```python
from build123d import *

# Parameters (mm, degrees)
FILLET1_R   = 0.2
HEX_2_DEPTH = 1.9


with BuildPart() as part:
    # BodySke → BaseBody (revolve)
    with BuildSketch(Plane.XY):
        Polygon((0, 0), (0, 4.715), (0.885, 4.715), (3.1, 2.5), (15.555, 2.5), (16, 2.055), (16, 0), align=None)
    revolve(axis=Axis((0, 0, 0), (1, 0, 0)))

    # Fillet1
    fillet1_edges = [part.edges().sort_by_distance(p)[0] for p in [
        (3.1, -2.5, 0),
    ]]
    fillet(fillet1_edges, radius=FILLET1_R)

    # Sketch2 → PreBroach (revolve, cut)
    with BuildSketch(Plane.XY):
        Polygon((0, 1.5), (1.9, 1.5), (2.766025404, 0), (0, 0), align=None)
    revolve(axis=Axis((0, 0, 0), (1, 0, 0)), mode=Mode.SUBTRACT)

    # Sketch3 → Hex 2 (cut)
    with BuildSketch(Plane.ZY):
        Polygon((-1.5, -0.866025404), (-1.5, 0.866025404), (0, 1.732050808), (1.5, 0.866025404), (1.5, -0.866025404), (0, -1.732050808), align=None)
    extrude(amount=-HEX_2_DEPTH, mode=Mode.SUBTRACT)


solid = part.part
```
Could you check a few things on this model? Use its own coordinates, in mm. A direction names the side the tool comes from. Coordinates: 2 decimals unless noted, no trailing zeros. Write each loop counter-clockwise with the first axis right and the second up, starting at its lowest first coordinate (ties: lowest second). Pieces come first, ordered by that corner, then holes. Notation, with made-up numbers: (7.25, -26) -> (30.25, -26) arc R32 cw to (30.25, 5) -> close; hole circle Ø10 at (-13, 35.25). An arc over 180 degrees is marked (long way). Write item = value, one per line. Start each with the question number.
(1) Will these pins go through, and if not, where does the flat tip stop? pin 1 (2 mm diameter, centred on x = 3.5, y = 3, fed in from +Z); pin 2 (3 mm diameter, centred on x = 8, z = -1.5, fed in from +Y); pin 3 (0.9 mm diameter, centred on x = 1.5, y = 0, fed in from -Z).
(2) Which directions (+Z, -Z, +X, -X, +Y, -Y) give clear straight access to the entire face, cutting with the end or side of a thin tool? Please do faces 4 (the face through (1, 0, -1.5)), 5 (the face through (9.456, 2.385, 0.751)), 6 (the face through (0, -2, 0)).
(3) I need wall thicknesses on line 1 (X direction, y = -0.5, z = 3); line 2 (Z direction, x = 3.5, y = -2); line 3 (Y direction, x = 15.25, z = 0). Which ranges of each line are inside material? Lowest first, please. Write a range as [from, to].
(4) I want a section at A-A (x = 3.5). Please give me the cut outline in (y, z).
(5) We'd pull the mould along Z, two halves only. Please class faces 1 (the face through (1, 0, 1.5)), 2 (the face through (16, 0, 0)), 3 (the face through (0.449, -0.614, 4.675)): released by +Z, released by -Z, zero draft, split by the parting line, or undercut.
Result set:
q1.pin_1 = 1.63
q1.pin_2 = 2.5
q1.pin_3 = -4.55
q2.face_4 = -X
q2.face_5 = +X
q2.face_6 = +Z, -Z, -X, +Y, -Y
q3.line_1 = [0, 2.56]
q3.line_2 = [-1.5, 1.5]
q3.line_3 = [-2.5, 2.5]
q4.outline = circle Ø5 at (0, 0)
q5.face_1 = undercut
q5.face_2 = zero draft
q5.face_3 = split by the parting line
